Can you work these out from the model? Positions are in its coordinate system, mm. A direction names the side the tool comes from. Coordinates: 2 decimals unless noted, no trailing zeros. Loops run counter-clockwise (first coordinate to the right, second up) from the corner with the lowest first, then second, coordinate; pieces in that order, holes last.
```python
from build123d import *

# Parameters (mm, degrees)
BOSS_EXTRUDE1_START = 123.5
SKETCH1_W           = 85
SKETCH1_H           = 44
BOSS_EXTRUDE1_DEPTH = 1.5
BOSS_EXTRUDE2_START = 14.1
SKETCH2_R           = 6.5
BOSS_EXTRUDE2_DEPTH = 2.1
BOSS_EXTRUDE3_START = 14.1
SKETCH3_W           = 14.3
SKETCH3_H           = 13
BOSS_EXTRUDE3_DEPTH = 2.1
CUT_EXTRUDE1_START  = 14.1
SKETCH4_R           = 3.55
CUT_EXTRUDE1_DEPTH  = 2.1
CUT_EXTRUDE2_START  = 14.1
CUT_EXTRUDE2_DEPTH  = 2.1
BOSS_EXTRUDE4_START = -24.5
SKETCH6_R           = 6.5
BOSS_EXTRUDE4_DEPTH = 1.5
BOSS_EXTRUDE5_START = -24.5
SKETCH7_W           = 14.3
SKETCH7_H           = 13
BOSS_EXTRUDE5_DEPTH = 1.5
CUT_EXTRUDE3_START  = -24.5
SKETCH8_R           = 2.95
CUT_EXTRUDE3_DEPTH  = 1.5


with BuildPart() as part:
    # Sketch1 → Boss-Extrude1 (new, symmetric)
    with BuildSketch(Plane(origin=(0, 0, 0), x_dir=(0, 0, -1), z_dir=(1, 0, 0)).offset(BOSS_EXTRUDE1_START)):
        with Locations((-4.5, 24)):
            Rectangle(SKETCH1_W, SKETCH1_H)
    extrude(amount=BOSS_EXTRUDE1_DEPTH, both=True)



with BuildPart() as body_2:
    # Sketch2 → Boss-Extrude2 (new, symmetric)
    with BuildSketch(Plane.XY.offset(BOSS_EXTRUDE2_START)):
        with Locations((108.2, 18.5)):
            Circle(SKETCH2_R)
    extrude(amount=BOSS_EXTRUDE2_DEPTH, both=True)


with BuildPart() as part_1:
    add(part.part)

    add(body_2.part)  # Boss-Extrude3 merges body 2
    # Sketch3 → Boss-Extrude3 (add, symmetric)
    with BuildSketch(Plane.XY.offset(BOSS_EXTRUDE3_START)):
        with Locations((115.35, 18.5)):
            Rectangle(SKETCH3_W, SKETCH3_H)
    extrude(amount=BOSS_EXTRUDE3_DEPTH, both=True)

    # Sketch4 → Cut-Extrude1 (cut, symmetric)
    with BuildSketch(Plane.XY.offset(CUT_EXTRUDE1_START)):
        with Locations((108.2, 18.5)):
            Circle(SKETCH4_R)
    extrude(amount=CUT_EXTRUDE1_DEPTH, both=True, mode=Mode.SUBTRACT)

    # Sketch5 → Cut-Extrude2 (cut, symmetric)
    with BuildSketch(Plane.XY.offset(CUT_EXTRUDE2_START)):
        Polygon((108.2, 14.95), (120.9, 16.096718595), (120.9, 20.903281405), (108.2, 22.05), align=None)
    extrude(amount=CUT_EXTRUDE2_DEPTH, both=True, mode=Mode.SUBTRACT)



with BuildPart() as body_2_2:
    # Sketch6 → Boss-Extrude4 (new, symmetric)
    with BuildSketch(Plane.XY.offset(BOSS_EXTRUDE4_START)):
        with Locations(Location((108.2, 18.5, 0), (0, 0, 180))):
            Circle(SKETCH6_R)
    extrude(amount=BOSS_EXTRUDE4_DEPTH, both=True)


with BuildPart() as part_2:
    add(part_1.part)

    add(body_2_2.part)  # Boss-Extrude5 merges body 2 2
    # Sketch7 → Boss-Extrude5 (add, symmetric)
    with BuildSketch(Plane.XY.offset(BOSS_EXTRUDE5_START)):
        with Locations((115.35, 18.5)):
            Rectangle(SKETCH7_W, SKETCH7_H)
    extrude(amount=BOSS_EXTRUDE5_DEPTH, both=True)

    # Sketch8 → Cut-Extrude3 (cut, symmetric)
    with BuildSketch(Plane.XY.offset(CUT_EXTRUDE3_START)):
        with Locations((108.2, 18.5)):
            Circle(SKETCH8_R)
    extrude(amount=CUT_EXTRUDE3_DEPTH, both=True, mode=Mode.SUBTRACT)


solid = part_2.part
```
(1) Which directions (+Z, -Z, +X, -X, +Y, -Y) give clear straight access to the entire face, cutting with the end or side of a thin tool? Please do faces 1 (the flat face through (115, 25, -24)), 2 (the flat face through (112, 18, -23)), 3 (the flat face through (112, 23, 16.2)), 4 (the flat face through (114.783, 15.544, 14.129)), 5 (the flat face through (115, 12, 14)).
Check values:
face 1: +Z, -Z, -X, +Y
face 2: -X, +Y, -Y
face 3: +Z, -X, +Y, -Y
face 4: +Z
face 5: +Z, -Z, -X, -Y
(2) I want a section at A-A on y = 18.5. Write out the boundary of the cut face in (x, z).
Check values:
outline: (101.7, -26) - (105.25, -26) - (105.25, -23) - (101.7, -23) - close; (101.7, 12) - (104.65, 12) - (104.65, 16.2) - (101.7, 16.2) - close; (111.15, -26) - (122, -26) - (122, -38) - (125, -38) - (125, 47) - (122, 47) - (122, 16.2) - (120.9, 16.2) - (120.9, 12) - (122, 12) - (122, -23) - (111.15, -23) - close
(3) If we mould it in two halves opening along X, with no side actions, what happens to faces 6 (the cylindrical face through (101.7, 18.6, 14.1)), 7 (the flat face through (114.95, 21.44, 14.13)), 8 (the flat face through (124, 2, 5))? For each: released by +X, released by -X, zero draft, split by the parting line, or undercut.
Check values:
face 6: released by -X
face 7: undercut
face 8: zero draft
(4) I want a section at B-B on x = 115.75. Write out the boundary of the cut face in (y, z).
Check values:
outline: (12, -26) - (25, -26) - (25, -23) - (12, -23) - close; (12, 12) - (15.63, 12) - (15.63, 16.2) - (12, 16.2) - close; (21.37, 12) - (25, 12) - (25, 16.2) - (21.37, 16.2) - close
(5) I want a section at C-C on z = 26. Write out the boundary of the cut face in (x, y), then the cut area to 3 significant figures.
Check values:
outline: (122, 2) - (125, 2) - (125, 46) - (122, 46) - close
area: 132 mm2
(6) If I drill on probe 1 along Y at (x, z) = (108.2, -25.1); probe 2 along X at (y, z) = (18.5, 14.9); probe 3 along X at (y, z) = (13.5, 1.5), over which ranges is the centre line in solid material (lowest first)?
Check values:
probe 1: y = 12 to 15.55, 21.45 to 25
probe 2: x = 101.7 to 104.65, 120.9 to 125
probe 3: x = 122 to 125
(7) I'm going to push flat-ended pins straight in: pin 1 (3 mm diameter, centred on y = 22, z = -10, fed in from -X); pin 2 (6.5 mm diameter, centred on x = 109, y = 20, fed in from -Z); pin 3 (2.5 mm diameter, centred on x = 118.5, z = -25, fed in from -Y). Where does each tip first touch, or does it pass through?
Check values:
pin 1: stops at x = 122
pin 2: stops at z = -26
pin 3: stops at y = 12
(8) I want a section at D-D on y = 35.5. Write out the boundary of the cut face in (x, z), then the cut area to 3 significant figures.
Check values:
outline: (122, -38) - (125, -38) - (125, 47) - (122, 47) - close
area: 255 mm2
